Can you work these out from the model? Positions are in its coordinate system, mm. Give positions to 0.01 mm unless a question says otherwise; leave off trailing zeros. Loops run counter-clockwise (first coordinate to the right, second up) from the corner with the lowest first, then second, coordinate; pieces in that order, holes last.
from build123d import *

# Parameters (mm, degrees)
CYLINDER043_R     = 1.38
CYLINDER043_DEPTH = 10
CYLINDER042_R     = 1.38
CYLINDER042_DEPTH = 10
BOX025_W          = 25
BOX025_H          = 10
BOX025_DEPTH      = 4
FILLET_R          = 3


with BuildPart() as cylinder043:
    # Cylinder043 → Cylinder043 (new body)
    with BuildSketch(Plane(origin=(25, 52, 59), x_dir=(1, 0, 0), z_dir=(0, 0, 1))):
        Circle(CYLINDER043_R)
    extrude(amount=CYLINDER043_DEPTH)


with BuildPart() as cylinder042:
    # Cylinder042 → Cylinder042 (new body)
    with BuildSketch(Plane(origin=(40, 52, 59), x_dir=(1, 0, 0), z_dir=(0, 0, 1))):
        Circle(CYLINDER042_R)
    extrude(amount=CYLINDER042_DEPTH)


with BuildPart() as fillet_body:
    # Box025 → Box025 (new body)
    with BuildSketch(Plane(origin=(45, 57, 62), x_dir=(-1, 0, 0), z_dir=(0, 0, 1))):
        with Locations((12.5, 5)):
            Rectangle(BOX025_W, BOX025_H)
    extrude(amount=BOX025_DEPTH)

    # Cut022: cut Cylinder042
    add(cylinder042.part, mode=Mode.SUBTRACT)

    # Cut023: cut Cylinder043
    add(cylinder043.part, mode=Mode.SUBTRACT)

    # Fillet
    fillet_edges = [fillet_body.edges().sort_by_distance(p)[0] for p in [
        (20, 57, 64),
        (20, 47, 64),
    ]]
    fillet(fillet_edges, radius=FILLET_R)


with BuildPart() as fillet_body_1:
    # Fillet placement: moved
    add(fillet_body.part.moved(Location((-2, 5, 0))))


solid = fillet_body_1.part
(1) Suppose I cut it at C-C on z = 64.7. List the corners of the cut face in (x, y) for me, plus the area to 3 significant figures.
Returned:
outline: (18, 55) arc R3 ccw to (21, 52) - (43, 52) - (43, 62) - (21, 62) arc R3 ccw to (18, 59) - close; hole circle Ø2.76 at (23, 57); hole circle Ø2.76 at (38, 57)
area: 234 mm2
(2) Suppose I cut it at A-A on y = 57. List the corners of the cut face in (x, z) for me, plus the area to 3 significant figures.
Returned:
outline: (18, 62) - (21.62, 62) - (21.62, 66) - (18, 66) - close; (24.38, 62) - (36.62, 62) - (36.62, 66) - (24.38, 66) - close; (39.38, 62) - (43, 62) - (43, 66) - (39.38, 66) - close
area: 77.9 mm2
(3) Please list where these lines run through material, in increasing order: probe 1 along X at (y, z) = (57, 64.6); probe 2 along Y at (x, z) = (38, 64.6); probe 3 along X at (y, z) = (56.25, 63.4).
Returned:
probe 1: x = 18 to 21.62, 24.38 to 36.62, 39.38 to 43
probe 2: y = 52 to 55.62, 58.38 to 62
probe 3: x = 18 to 21.84, 24.16 to 36.84, 39.16 to 43
(4) Thinking about a two-plate mould opening in Y: for faces 1 (the cylindrical face through (36.62, 57.06, 63.97)), 2 (the flat face through (32, 62, 64)), 3 (the cylindrical face through (18.9, 52.86, 64.03)), which applies, pulls with the +Y half, pulls with the -Y half, needs draft (parallel to the pull), parting line crosses it, or undercut?
Returned:
face 1: undercut
face 2: pulls with the +Y half
face 3: pulls with the -Y half
(5) Suppose I cut it at B-B on x = 23. List the corners of the cut face in (y, z) for me.
Returned:
outline: (52, 62) - (55.62, 62) - (55.62, 66) - (52, 66) - close; (58.38, 62) - (62, 62) - (62, 66) - (58.38, 66) - close
(6) Suppose I cut it at D-D on y = 58. List the corners of the cut face in (x, z) for me.
Returned:
outline: (18, 62) - (22.05, 62) - (22.05, 66) - (18, 66) - close; (23.95, 62) - (37.05, 62) - (37.05, 66) - (23.95, 66) - close; (38.95, 62) - (43, 62) - (43, 66) - (38.95, 66) - close
